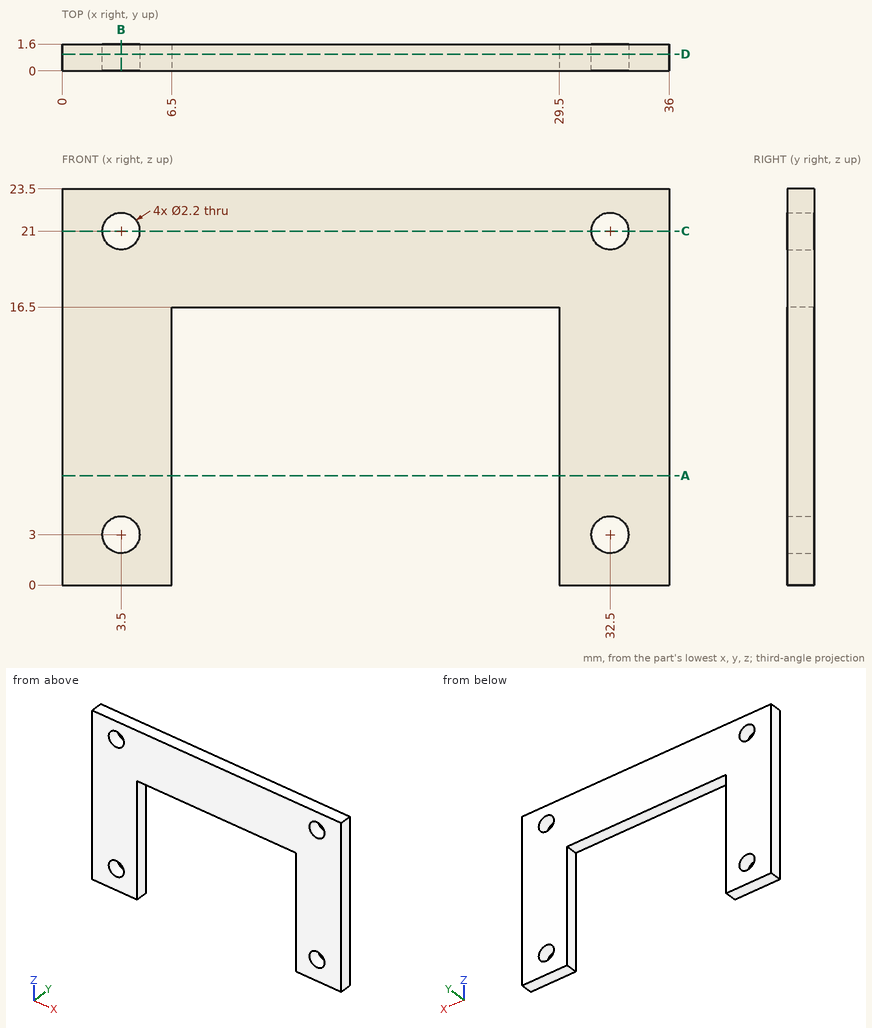
Geometry: see drawing. Coordinates: mm, zero at the bounding-box minimum. Coordinates: 2 decimals unless noted, no trailing zeros. Loops run counter-clockwise (first coordinate to the right, second up) from the corner with the lowest first, then second, coordinate; pieces in that order, holes last. Notation, with made-up numbers: M -15.5,53.5 L -11.5,53.5 A25 cw -11.5,73.5 Z; hole C 24.25,71 d2. An arc over 180 degrees is marked long. Answer in a Markdown table with one row per item.
Q1. Ray query, probe 1 along X at (y, z) = (0.6, 21); probe 2 along Z at (x, y) = (3.5, 0.55); probe 3 along X at (y, z) = (1.3, 3). Return the intervals inside material, ascending. Write a range as from..to.
Answers below:
| item | result |
|---|---|
| probe 1 | x = 0..2.4, 4.6..31.4, 33.6..36 |
| probe 2 | z = 0..1.9, 4.1..19.9, 22.1..23.5 |
| probe 3 | x = 0..2.4, 4.6..6.5, 29.5..31.4, 33.6..36 |
Q2. Section C-C on z = 21. Return the cut outline in (x, y).
Answers below:
| item | result |
|---|---|
| outline | M 0,0 L 2.4,0 L 2.4,1.6 L 0,1.6 Z; M 4.6,0 L 31.4,0 L 31.4,1.6 L 4.6,1.6 Z; M 33.6,0 L 36,0 L 36,1.6 L 33.6,1.6 Z |
Q3. First-contact query: pin 1 (2.5 mm diameter, centred on x = 32.5, z = 3, fed in from -Y); pin 2 (0.8 mm diameter, centred on x = 22.5, y = 0.5, fed in from -Z). Flat tips, straight axial feed; report the tip coordinate or a pass-through.
Answers below:
| item | result |
|---|---|
| pin 1 | stops at y = 0 |
| pin 2 | stops at z = 16.5 |
Q4. Section B-B on x = 3.5. Return the cut outline in (y, z).
Answers below:
| item | result |
|---|---|
| outline | M 0,0 L 1.6,0 L 1.6,1.9 L 0,1.9 Z; M 0,4.1 L 1.6,4.1 L 1.6,19.9 L 0,19.9 Z; M 0,22.1 L 1.6,22.1 L 1.6,23.5 L 0,23.5 Z |
Q5. Section A-A on z = 6.5. Return the cut outline in (x, y), plus the area to 3 significant figures.
Answers below:
| item | result |
|---|---|
| outline | M 0,0 L 6.5,0 L 6.5,1.6 L 0,1.6 Z; M 29.5,0 L 36,0 L 36,1.6 L 29.5,1.6 Z |
| area | 20.8 mm^2 |
Q6. Section D-D on y = 1. Return the cut outline in (x, z).
Answers below:
| item | result |
|---|---|
| outline | M 0,0 L 6.5,0 L 6.5,16.5 L 29.5,16.5 L 29.5,0 L 36,0 L 36,23.5 L 0,23.5 Z; hole C 3.5,3 d2.2; hole C 3.5,21 d2.2; hole C 32.5,3 d2.2; hole C 32.5,21 d2.2 |
